```python
from build123d import *

# Parameters (mm, degrees)
SM_BASE_FLANGE_1_DEPTH = 27.5
CHAMFER_1_SIZE         = 4
SKETCH_6_R             = 9.5
CUT_EXTRUDE_1_DEPTH    = 62.386073339
SKETCH_7_W             = 12
SKETCH_7_H             = 23
CUT_EXTRUDE_2_DEPTH    = 62.386073339
CHAMFER_2_SIZE         = 2
SKETCH_9_W             = 23
SKETCH_9_H             = 10.5
CUT_EXTRUDE_4_DEPTH    = 62.386073339
CUT_EXTRUDE_5_REACH    = 63.386
SKETCH_10_R            = 1.65


# Sheet-metal steps are written as plain solids
with BuildPart() as part:
    # Sketch 1 → 基材-凸緣1 (new, symmetric)
    with BuildSketch(Plane(origin=(0, 0, 0), x_dir=(0, 1, 0), z_dir=(-1, 0, 0))):
        with BuildLine():
            Line((-50, 0), (-1.242640687, 0))
            ThreePointArc((-1.242640687, 0), (-0.09459039, -0.228361402), (0.878679656, -0.878679656))
            Line((0.878679656, -0.878679656), (21.213203436, -21.213203436))
            Line((21.213203436, -21.213203436), (19.798989873, -22.627416998))
            Line((19.798989873, -22.627416998), (-0.535533906, -2.292893219))
            ThreePointArc((-0.535533906, -2.292893219), (-0.859957255, -2.076120467), (-1.242640687, -2))
            Line((-1.242640687, -2), (-50, -2))
            Line((-50, -2), (-50, 0))
        make_face()
    extrude(amount=SM_BASE_FLANGE_1_DEPTH, both=True)

    # 導角1
    chamfer_1_edges = [part.edges().sort_by_distance(p)[0] for p in [
        (-27.5, -50, 1),
        (-27.5, 20.506096654, 21.920310217),
        (27.5, -50, 1),
        (27.5, 20.506096654, 21.920310217),
    ]]
    chamfer(chamfer_1_edges, length=CHAMFER_1_SIZE)

    # 草圖6 → 除料-伸長1 (cut, through all)
    with BuildSketch(Plane(origin=(0, 0, 0), x_dir=(-0.9655064458746985, -0.1841158643007276, -0.18411586430072824), z_dir=(0, 0.7071067811865488, -0.7071067811865465))):
        with Locations(Location((-4.42644559, 16.41360958, 0), (0, 0, 105.092560886))):
            Circle(SKETCH_6_R)
    extrude(amount=-CUT_EXTRUDE_1_DEPTH, mode=Mode.SUBTRACT)

    # 草圖7 → 除料-伸長2 (cut, through all)
    with BuildSketch(Plane(origin=(0, 0, 0), x_dir=(-1, 0, 0), z_dir=(0, 0, -1))):
        with Locations((-21.5, -27)):
            Rectangle(SKETCH_7_W, SKETCH_7_H)
    cut_extrude_2 = extrude(amount=-CUT_EXTRUDE_2_DEPTH, mode=Mode.SUBTRACT)

    # 鏡射1: 除料-伸長2 across plane
    add(cut_extrude_2.mirror(Plane(origin=(0, 0, 0), x_dir=(0, 0, 1), z_dir=(1, 0, 0))), mode=Mode.SUBTRACT)

    # 導角2
    chamfer_2_edges = [part.edges().sort_by_distance(p)[0] for p in [
        (-15.5, -38.5, 1),
        (-15.5, -15.5, 1),
        (27.5, -38.5, 1),
        (27.5, -15.5, 1),
        (15.5, -15.5, 1),
        (15.5, -38.5, 1),
        (-27.5, -15.5, 1),
        (-27.5, -38.5, 1),
    ]]
    chamfer(chamfer_2_edges, length=CHAMFER_2_SIZE)

    # 草圖9 → 除料-伸長4 (cut, through all)
    with BuildSketch(Plane(origin=(0, 0, 0), x_dir=(-1, 0, 0), z_dir=(0, 0, -1))):
        with Locations((0, -15)):
            Rectangle(SKETCH_9_W, SKETCH_9_H)
    extrude(amount=-CUT_EXTRUDE_4_DEPTH, mode=Mode.SUBTRACT)

    # 草圖10 → 除料-伸長5 (cut, up to next)
    with BuildSketch(Plane(origin=(0, 0, 0), x_dir=(-1, 0, 0), z_dir=(0, 0, -1)), mode=Mode.PRIVATE) as cut_extrude_5_sk1:
        with Locations((20, -45)):
            Circle(SKETCH_10_R)
    cut_extrude_5_tool1 = extrude(cut_extrude_5_sk1.sketch, amount=-CUT_EXTRUDE_5_REACH, mode=Mode.PRIVATE) & part.part
    # 草圖10 → 除料-伸長5 (cut, up to next)
    with BuildSketch(Plane(origin=(0, 0, 0), x_dir=(-1, 0, 0), z_dir=(0, 0, -1)), mode=Mode.PRIVATE) as cut_extrude_5_sk2:
        with Locations((-20, -45)):
            Circle(SKETCH_10_R)
    cut_extrude_5_tool2 = extrude(cut_extrude_5_sk2.sketch, amount=-CUT_EXTRUDE_5_REACH, mode=Mode.PRIVATE) & part.part
    # 草圖10 → 除料-伸長5 (cut, up to next)
    with BuildSketch(Plane(origin=(0, 0, 0), x_dir=(-1, 0, 0), z_dir=(0, 0, -1)), mode=Mode.PRIVATE) as cut_extrude_5_sk3:
        with Locations((-20, -5)):
            Circle(SKETCH_10_R)
    cut_extrude_5_tool3 = extrude(cut_extrude_5_sk3.sketch, amount=-CUT_EXTRUDE_5_REACH, mode=Mode.PRIVATE) & part.part
    # 草圖10 → 除料-伸長5 (cut, up to next)
    with BuildSketch(Plane(origin=(0, 0, 0), x_dir=(-1, 0, 0), z_dir=(0, 0, -1)), mode=Mode.PRIVATE) as cut_extrude_5_sk4:
        with Locations((20, -5)):
            Circle(SKETCH_10_R)
    cut_extrude_5_tool4 = extrude(cut_extrude_5_sk4.sketch, amount=-CUT_EXTRUDE_5_REACH, mode=Mode.PRIVATE) & part.part
    add(cut_extrude_5_tool1.solids().sort_by_distance((-20, -45, 0))[0], mode=Mode.SUBTRACT)
    add(cut_extrude_5_tool2.solids().sort_by_distance((20, -45, 0))[0], mode=Mode.SUBTRACT)
    add(cut_extrude_5_tool3.solids().sort_by_distance((20, -5, 0))[0], mode=Mode.SUBTRACT)
    add(cut_extrude_5_tool4.solids().sort_by_distance((-20, -5, 0))[0], mode=Mode.SUBTRACT)


solid = part.part
```
Check sheet for the modelled part. Datum: model origin and axes. Units: mm. A direction names the side the tool comes from. Coordinates: 2 decimals unless noted, no trailing zeros. Loops run counter-clockwise (first coordinate to the right, second up) from the corner with the lowest first, then second, coordinate; pieces in that order, holes last. Notation, with made-up numbers: M -2,10.5 L 24,10.5 A35 ccw 24,49.5 Z; hole C 23,2.25 d9. An arc over 180 degrees is marked long. Answer as a JSON object with one key per item and string values.
1. Access from +Z, -Z, +X, -X, +Y, -Y to the whole of each face (thin tool, end or side, straight path). Record for faces 4 (the flat face through (0, -25, 2)), 5 (the flat face through (11.5, -15, 1)), 6 (the flat face through (16, -17, 1)), 7 (the flat face through (27.5, 4, 6)), 8 (the flat face through (-22, -15.5, 1)).
Outcome:
{"face 4": "+Z, +X, -X, -Y", "face 5": "+Z, -Z", "face 6": "+Z, -Z, +X", "face 7": "+Z, -Z, +X, +Y, -Y", "face 8": "+Z, -Z, -X"}
2. Scan lines: L1, parallel to Y at x = 20, z = 0.8; L2, parallel to Z at x = 11.5, y = -46; L3, parallel to Y at x = -20, z = 0.6. Record each from-to range of solid material in increasing order. Write a range as from..to.
Outcome:
{"L1": "-50..-46.65, -43.35..-38.5, -15.5..-6.65, -3.35..0.8", "L2": "0..2", "L3": "-50..-46.65, -43.35..-38.5, -15.5..-6.65, -3.35..0.56"}
3. Release check for a two-part mould opening along X. For faces 1 (the flat face through (-25.5, 19.1, 20.5)), 2 (the flat face through (0, -20.25, 1)), 3 (the flat face through (22, -38.5, 1)) record: pulls with the +X half, pulls with the -X half, needs draft (parallel to the pull), parting line crosses it, or undercut.
Outcome:
{"face 1": "pulls with the -X half", "face 2": "undercut", "face 3": "needs draft"}
4. Sectioned sample at C-C on x = -1.5. Record the cut outline in (y, z), and give its area (3 significant figures).
Outcome:
{"outline": "M -50,0 L -20.25,0 L -20.25,2 L -50,2 Z; M -9.75,0 L -1.24,0 A3 ccw 0.88,0.88 L 5.39,5.39 L 3.97,6.8 L -0.54,2.29 A1 cw -1.24,2 L -9.75,2 Z; M 17.24,20.07 L 18.65,18.65 L 21.21,21.21 L 19.8,22.63 Z", "area": "99.6 mm²"}
5. Sectioned sample at A-A on y = -45. Record the cut outline in (x, z).
Outcome:
{"outline": "M -27.5,0 L -21.65,0 L -21.65,2 L -27.5,2 Z; M -18.35,0 L 18.35,0 L 18.35,2 L -18.35,2 Z; M 21.65,0 L 27.5,0 L 27.5,2 L 21.65,2 Z"}
6. Depth check by flat-ended pin: P1, Ø6, axis at x = -14.5, y = -25.5, coming from the +Z side; P2, Ø3, axis at x = 20, y = -5, coming from the +Z side; P3, Ø1.6, axis at x = -19.5, z = 1, coming from the +Y side; P4, Ø4, axis at x = -8, z = 13.5, coming from the +Y side. Enter the tip coordinate at first touch or a pass-through.
Outcome:
{"P1": "z = 2", "P2": "through", "P3": "y = 1.8", "P4": "y = 15.5"}
7. Sectioned sample at B-B on x = 20. Record the cut outline in (y, z), and give its area (3 significant figures).
Outcome:
{"outline": "M -50,0 L -46.65,0 L -46.65,2 L -50,2 Z; M -43.35,0 L -38.5,0 L -38.5,2 L -43.35,2 Z; M -15.5,0 L -6.65,0 L -6.65,2 L -15.5,2 Z; M -3.35,0 L -1.24,0 A3 ccw 0.88,0.88 L 21.21,21.21 L 19.8,22.63 L -0.54,2.29 A1 cw -1.24,2 L -3.35,2 Z", "area": "99.0 mm²"}
8. Sectioned sample at D-D on y = -27.5. Record the cut outline in (x, z), and give its area (3 significant figures).
Outcome:
{"outline": "M -15.5,0 L 15.5,0 L 15.5,2 L -15.5,2 Z", "area": "62.0 mm²"}
